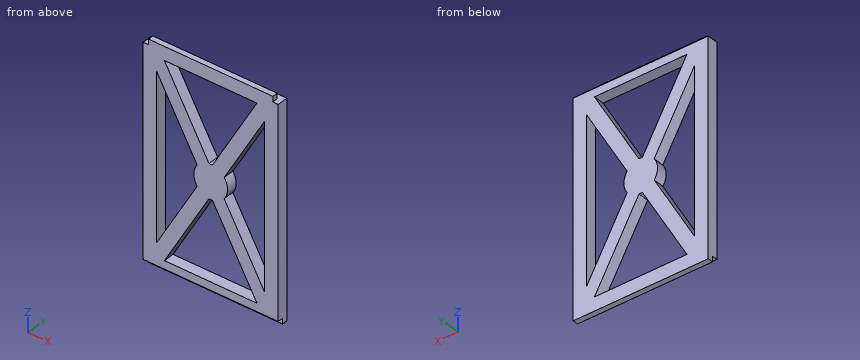
from build123d import *

# Parameters (mm, degrees)
F0_W     = 100
F0_H     = 161.8
F1_DEPTH = 8
F2_W     = 4
F2_H     = 4
F3_DEPTH = 134.44841
F4_W     = 4
F4_H     = 4
F5_DEPTH = 4


with BuildPart() as f1:
    # F0 (on Front) → F1 (new body)
    with BuildSketch(Plane.XZ):
        with Locations((50, 80.9)):
            Rectangle(F0_W, F0_H)
        with BuildLine():
            Line((84.259152, 10), (15.740848, 10))
            Line((15.740848, 10), (48.725419, 68.465152))
            ThreePointArc((48.725419, 68.465152), (50, 68.4), (51.274581, 68.465152))
            Line((51.274581, 68.465152), (84.259152, 10))
        make_face(mode=Mode.SUBTRACT)
        with BuildLine():
            Line((40.015904, 73.378842), (10, 20.175653))
            Line((10, 20.175653), (10, 141.624347))
            Line((10, 141.624347), (40.015904, 88.421158))
            ThreePointArc((40.015904, 88.421158), (37.5, 80.9), (40.015904, 73.378842))
        make_face(mode=Mode.SUBTRACT)
        with BuildLine():
            Line((90, 141.624347), (90, 20.175653))
            Line((90, 20.175653), (59.984096, 73.378842))
            ThreePointArc((59.984096, 73.378842), (62.5, 80.9), (59.984096, 88.421158))
            Line((59.984096, 88.421158), (90, 141.624347))
        make_face(mode=Mode.SUBTRACT)
        with BuildLine():
            Line((15.740848, 151.8), (84.259152, 151.8))
            Line((84.259152, 151.8), (51.274581, 93.334848))
            ThreePointArc((51.274581, 93.334848), (50, 93.4), (48.725419, 93.334848))
            Line((48.725419, 93.334848), (15.740848, 151.8))
        make_face(mode=Mode.SUBTRACT)
    extrude(amount=F1_DEPTH)

    # F2 (on face) → F3 (cut)
    with BuildSketch(Plane(origin=(0, 0, 0), x_dir=(0, -1, 0), z_dir=(-1, 0, 0))):
        with Locations((2, 159.8)):
            Rectangle(F2_W, F2_H)
        with Locations((6, 2)):
            Rectangle(F2_W, F2_H)
    extrude(amount=-F3_DEPTH, mode=Mode.SUBTRACT)

    # F4 (on face) → F5 (cut)
    with BuildSketch(Plane.XY.offset(161.8)):
        with Locations((98, -6)):
            Rectangle(F4_W, F4_H)
        with Locations((2, -6)):
            Rectangle(F4_W, F4_H)
    extrude(amount=-F5_DEPTH, mode=Mode.SUBTRACT)


solid = f1.part
Input: part model. Units: mm. Frame: model coordinates. Give positions to 0.01 mm unless a question says otherwise; leave off trailing zeros. Write each loop counter-clockwise with the first axis right and the second up, starting at its lowest first coordinate (ties: lowest second). Pieces come first, ordered by that corner, then holes.
Q1. Section C-C, the plane x = 6. Output: boundary loops of the cut face in (y, z).
Q2. Material intervals for probe 1 along X at (y, z) = (-7.25, 41.5); probe 2 along Z at (x, y) = (69, -2); probe 3 along Z at (x, y) = (23.5, -3.5), sorted ascending.
Q3. Section B-B, the plane z = 149.5. Output: boundary loops of the cut face in (x, y).
Q4. Section D-D, the plane z = 113.5. Output: boundary loops of the cut face in (x, y).
Q5. First-contact query: P1, Ø2, axis at y = -7, z = 160, coming from the +X side; P2, Ø2, axis at y = -6.5, z = 160, coming from the -X side; P3, Ø1.2, axis at x = 55.5, z = 160.5, coming from the +Y side. Flat tips, straight axial feed; report the tip coordinate or a pass-through.
Q6. Section A-A, the plane x = 45. Output: boundary loops of the cut face in (y, z).
Filled in:
1. outline: (-8, 4) - (-4, 4) - (-4, 0) - (0, 0) - (0, 157.8) - (-4, 157.8) - (-4, 161.8) - (-8, 161.8) - close
2. probe 1: x = 0 to 10, 22.03 to 33.51, 66.49 to 77.97, 90 to 100
2. probe 2: z = 0 to 10, 37.05 to 57.4, 104.4 to 124.75, 151.8 to 157.8
2. probe 3: z = 0 to 10, 23.75 to 44.1, 117.7 to 138.05, 151.8 to 157.8
3. outline: (0, -8) - (17.04, -8) - (17.04, 0) - (0, 0) - close; (82.96, -8) - (100, -8) - (100, 0) - (82.96, 0) - close
4. outline: (0, -8) - (10, -8) - (10, 0) - (0, 0) - close; (25.87, -8) - (37.35, -8) - (37.35, 0) - (25.87, 0) - close; (62.65, -8) - (74.13, -8) - (74.13, 0) - (62.65, 0) - close; (90, -8) - (100, -8) - (100, 0) - (90, 0) - close
5. P1: stops at x = 96
5. P2: stops at x = 4
5. P3: stops at y = -4
6. outline: (-8, 4) - (-4, 4) - (-4, 0) - (0, 0) - (0, 10) - (-8, 10) - close; (-8, 61.86) - (0, 61.86) - (0, 99.94) - (-8, 99.94) - close; (-8, 151.8) - (0, 151.8) - (0, 157.8) - (-4, 157.8) - (-4, 161.8) - (-8, 161.8) - close
